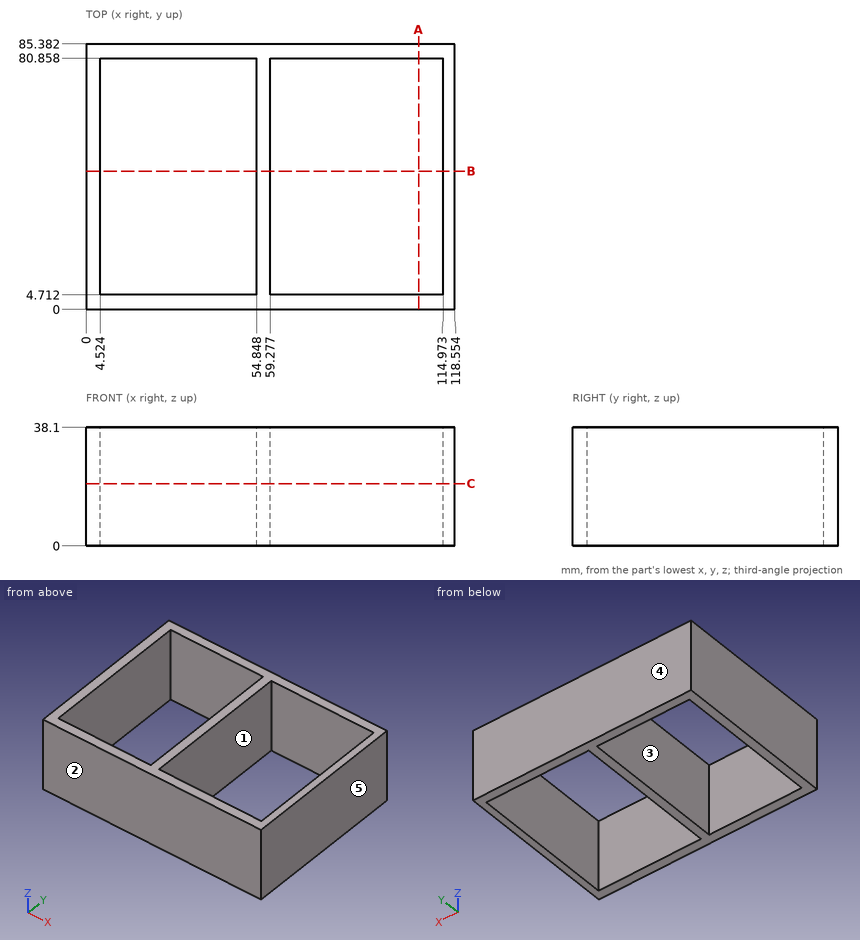
The figure shows three views and two pictorial views of one solid part (mm, origin at its lowest corner). Answer the questions. A direction names the side the tool comes from. Round coordinates to 2 decimals unless told otherwise and drop trailing zeros. Order: outer loops, then holes, each group sorted by start corner. A loop starts at its lowest first (then second) coordinate and runs counter-clockwise, first axis right, second up. Notation, with made-up numbers: (57, 86.5) -> (84, 86.5) arc R21 ccw to (84, 103.5) -> close; hole circle Ø11 at (-27, 70). An arc over 180 degrees is marked (long way). Put each result on its own line as item: value.
Q1. Section A-A, the plane x = 107 is taken. Write down the section's boundary in (y, z).
Results list:
outline: (0, 0) -> (4.71, 0) -> (4.71, 38.1) -> (0, 38.1) -> close; (80.86, 0) -> (85.38, 0) -> (85.38, 38.1) -> (80.86, 38.1) -> close
Q2. This flat-tipped pin is pushed along its axis until it touches: P1, Ø3, axis at x = 76, z = 14, coming from the -Y side. Where does it stop, or does it pass through?
Results list:
P1: y = 0
Q3. Consider line 1 along X through (y, z) = (22, 3.5) (1 decimal); line 2 along Y through (x, z) = (112, 18.5). Determine where each line is inside the solid, lowest interval first.
Results list:
line 1: 0 to 4.5, 54.8 to 59.3, 115 to 118.6
line 2: 0 to 4.71, 80.86 to 85.38
Q4. Section B-B, the plane y = 44.5 is taken. Write down the section's boundary in (x, z) (1 decimal).
Results list:
outline: (0, 0) -> (4.5, 0) -> (4.5, 38.1) -> (0, 38.1) -> close; (54.8, 0) -> (59.3, 0) -> (59.3, 38.1) -> (54.8, 38.1) -> close; (115, 0) -> (118.6, 0) -> (118.6, 38.1) -> (115, 38.1) -> close
Q5. Which of the six approach directions +Z, -Z, +X, -X, +Y, -Y give full straight-line access (tool end or side, diameter ignored) to the marked faces 1 and 2?
Results list:
face 1: +Z, -Z
face 2: +Z, -Z, +X, -X, -Y
Q6. Section C-C, the plane z = 20 is taken. Write down the section's boundary in (x, y) (1 decimal), and give its area (3 significant figures).
Results list:
outline: (0, 0) -> (118.6, 0) -> (118.6, 85.4) -> (0, 85.4) -> close; hole (4.5, 4.7) -> (54.8, 4.7) -> (54.8, 80.9) -> (4.5, 80.9) -> close; hole (59.3, 4.7) -> (115, 4.7) -> (115, 80.9) -> (59.3, 80.9) -> close
area: 2,050 mm^2
Q7. Determine the mould class of the marked faces 3, 4 and 5 for opening direction X: pulls with the +X half, pulls with the -X half, needs draft (parallel to the pull), parting line crosses it, or undercut.
Results list:
face 3: undercut
face 4: needs draft
face 5: pulls with the +X half
